Geometry check sheet. Reference: the model listing, model coordinates, mm. A direction names the side the tool comes from. Coordinates: 2 decimals unless noted, no trailing zeros. Loops run counter-clockwise (first coordinate to the right, second up) from the corner with the lowest first, then second, coordinate; pieces in that order, holes last. Notation, with made-up numbers: (-24, 44.25) - (5, 44.25) arc R17 cw to (5, 72.25) - close; hole circle Ø11 at (67, -4.75). An arc over 180 degrees is marked (long way). One line per item, written item: value.
from build123d import *

# Parameters (mm, degrees)
SKETCH_1_R          = 12.5
EXTRUDE_1_DEPTH     = 7.5
EXTRUDE_2_DEPTH     = 10
EXTRUDE_START       = -3
SKETCH_3_R          = 17
SKETCH_3_R_2        = 12.5
EXTRUDE_3_DEPTH     = 3
SKETCH_4_R          = 2.1000000000000005
CUT_EXTRUDE_1_DEPTH = 37.83761664386012
SKETCH_5_R          = 1.6000000000000003
CUT_EXTRUDE_2_DEPTH = 37.83761664386012
CUT_EXTRUDE_START   = -10
CUT_EXTRUDE_3_DEPTH = 10
SKETCH_7_R          = 17
SKETCH_7_R_2        = 12.500000000000004
EXTRUDE_4_DEPTH     = 0.5
SKETCH_8_R          = 15
SKETCH_8_R_2        = 12.499999999999996
EXTRUDE_5_DEPTH     = 11.5


# Read off the part's stored shape, not the designer's step: 凸台-拉伸2
with BuildPart() as part:
    # 草图1 → 凸台-拉伸1 (new, symmetric)
    with BuildSketch(Plane(origin=(0, 0, 0), x_dir=(1, 0, 0), z_dir=(0, 1, 0))):
        with Locations(Location((-1.39e-15, 1.39e-15, 0), (0, 0, 270))):
            Circle(SKETCH_1_R)
        with BuildLine():
            Line((6.600000000000003, -7.6000000000000005), (-6.599999999999996, -7.6000000000000005))
            ThreePointArc((-6.599999999999996, -7.6000000000000005), (-8.30710678118655, -8.307106781186542), (-7.599999999999978, -6.6000000000000005))
            Line((-7.599999999999996, -6.6000000000000005), (-7.599999999999996, 6.599999999999999))
            ThreePointArc((-7.599999999999978, 6.599999999999999), (-8.30710678118655, 8.30710678118654), (-6.599999999999996, 7.599999999999999))
            Line((-6.599999999999996, 7.599999999999999), (6.600000000000003, 7.599999999999999))
            ThreePointArc((6.600000000000002, 7.599999999999999), (7.600000000000003, 8.6), (8.600000000000005, 7.599999999999999))
            ThreePointArc((8.600000000000005, 7.599999999999999), (8.307106781186558, 6.892893218813457), (7.600000000000021, 6.599999999999998))
            Line((7.600000000000003, 6.599999999999999), (7.600000000000003, -6.6))
            ThreePointArc((7.600000000000021, -6.6), (8.307106781186558, -6.892893218813459), (8.600000000000003, -7.6000000000000005))
            ThreePointArc((8.600000000000003, -7.6000000000000005), (7.600000000000003, -8.600000000000001), (6.600000000000002, -7.6000000000000005))
        make_face(mode=Mode.SUBTRACT)
    extrude(amount=EXTRUDE_1_DEPTH, both=True)

    # 凸台-拉伸2 outline → 凸台-拉伸2 (add)
    with BuildSketch(Plane.XZ.offset(7.5)):
        with BuildLine():
            Line((10.6, -6.62495283), (10.6, 6.62495283))
            ThreePointArc((10.6, 6.62495283), (8.838834765, 8.838834765), (6.62495283, 10.6))
            Line((6.62495283, 10.6), (-6.62495283, 10.6))
            ThreePointArc((-6.62495283, 10.6), (-8.838834765, 8.838834765), (-10.6, 6.62495283))
            Line((-10.6, 6.62495283), (-10.6, -6.62495283))
            ThreePointArc((-10.6, -6.62495283), (-8.838834765, -8.838834765), (-6.62495283, -10.6))
            Line((-6.62495283, -10.6), (6.62495283, -10.6))
            ThreePointArc((6.62495283, -10.6), (8.838834765, -8.838834765), (10.6, -6.62495283))
        make_face()
        with BuildLine():
            ThreePointArc((-6.6, -7.6), (-8.307106781, -8.307106781), (-7.6, -6.6))
            Line((-7.6, -6.6), (-7.6, 6.6))
            ThreePointArc((-7.6, 6.6), (-8.307106781, 8.307106781), (-6.6, 7.6))
            Line((-6.6, 7.6), (6.6, 7.6))
            ThreePointArc((6.6, 7.6), (8.307106781, 8.307106781), (7.6, 6.6))
            Line((7.6, 6.6), (7.6, -6.6))
            ThreePointArc((7.6, -6.6), (8.307106781, -8.307106781), (6.6, -7.6))
            Line((6.6, -7.6), (-6.6, -7.6))
        make_face(mode=Mode.SUBTRACT)
    extrude_2 = extrude(amount=EXTRUDE_2_DEPTH)

    # 镜向1: 凸台-拉伸2 across plane
    add(extrude_2.mirror(Plane.ZX))

    # 草图3 → 凸台-拉伸3 (add)
    with BuildSketch(Plane.XZ.offset(7.5).offset(EXTRUDE_START)):
        with Locations(Location((0, 0, 0), (0, 0, 270))):
            Circle(SKETCH_3_R)
        with Locations(Location((0, 0, 0), (0, 0, 270))):
            Circle(SKETCH_3_R_2, mode=Mode.SUBTRACT)
    extrude(amount=EXTRUDE_3_DEPTH)

    # 草图4 → 切除-拉伸1 (cut, through all)
    with BuildSketch(Plane.XY.offset(10.600000000000001)):
        with Locations((-8.7e-16, -12.5)):
            Circle(SKETCH_4_R)
    extrude(amount=-CUT_EXTRUDE_1_DEPTH, mode=Mode.SUBTRACT)

    # 草图5 → 切除-拉伸2 (cut, through all)
    with BuildSketch(Plane(origin=(10.6, 0, 0), x_dir=(0, 0, -1), z_dir=(1, 0, 0))):
        with Locations((1.73e-15, 12.5)):
            Circle(SKETCH_5_R)
    extrude(amount=-CUT_EXTRUDE_2_DEPTH, mode=Mode.SUBTRACT)

    # 草图6 → 切除-拉伸3 (cut)
    with BuildSketch(Plane.XZ.offset(17.5).offset(CUT_EXTRUDE_START)):
        with BuildLine():
            Line((10.599999999999996, -6.624952830020757), (10.6, 6.624952830020752))
            ThreePointArc((10.6, 6.624952830020752), (8.83883476483184, 8.838834764831846), (6.6249528300207485, 10.600000000000001))
            Line((6.6249528300207485, 10.600000000000001), (-6.624952830020753, 10.600000000000001))
            ThreePointArc((-6.624952830020753, 10.600000000000001), (-8.838834764831846, 8.838834764831844), (-10.6, 6.624952830020758))
            Line((-10.6, 6.624952830020758), (-10.6, -6.624952830020761))
            ThreePointArc((-10.6, -6.624952830020761), (-8.83883476483185, -8.838834764831843), (-6.624952830020767, -10.599999999999994))
            Line((-6.624952830020767, -10.599999999999994), (6.624952830020759, -10.599999999999998))
            ThreePointArc((6.624952830020759, -10.599999999999998), (8.838834764831844, -8.838834764831844), (10.599999999999996, -6.624952830020757))
        make_face()
    extrude(amount=CUT_EXTRUDE_3_DEPTH, mode=Mode.SUBTRACT)

    # 草图7 → 凸台-拉伸4 (add)
    with BuildSketch(Plane(origin=(0, -4.5, 0), x_dir=(1, 0, 0), z_dir=(0, 1, 0))):
        with Locations(Location((0, 0, 0), (0, 0, 90))):
            Circle(SKETCH_7_R)
        with Locations(Location((0, 0, 0), (0, 0, 122.005199861))):
            Circle(SKETCH_7_R_2, mode=Mode.SUBTRACT)
    extrude(amount=EXTRUDE_4_DEPTH)

    # 草图8 → 凸台-拉伸5 (add)
    with BuildSketch(Plane(origin=(0, -4, 0), x_dir=(1, 0, 0), z_dir=(0, 1, 0))):
        with Locations(Location((0, 0, 0), (0, 0, 270))):
            Circle(SKETCH_8_R)
        Circle(SKETCH_8_R_2, mode=Mode.SUBTRACT)
    extrude(amount=EXTRUDE_5_DEPTH)


solid = part.part
(1) Release check for a two-part mould opening along Z. For faces 5 (the face through (9.121, 14.086, 0.208)), 6 (the face through (8.87, 12.43, 8.81)), 7 (the face through (0, -7.5, 8)) record: pulls with the +Z half, pulls with the -Z half, needs draft (parallel to the pull), parting line crosses it, or undercut.
Reply:
face 5: undercut
face 6: pulls with the +Z half
face 7: needs draft
(2) Cross-section at C-C on z = 2.5. Record the cut outline in (x, y).
Reply:
outline: (-16.82, -7.5) - (-7.6, -7.5) - (-7.6, 17.5) - (-10.6, 17.5) - (-10.6, 7.5) - (-14.79, 7.5) - (-14.79, -4) - (-16.82, -4) - close; (7.6, -7.5) - (16.82, -7.5) - (16.82, -4) - (14.79, -4) - (14.79, 7.5) - (10.6, 7.5) - (10.6, 17.5) - (7.6, 17.5) - close
(3) Cross-section at A-A on x = 0. Record the cut outline in (y, z).
Reply:
outline: (-7.5, -17) - (-4, -17) - (-4, -15) - (7.5, -15) - (7.5, -10.6) - (17.5, -10.6) - (17.5, -7.6) - (-7.5, -7.6) - close; (-7.5, 7.6) - (17.5, 7.6) - (17.5, 10.6) - (7.5, 10.6) - (7.5, 15) - (-4, 15) - (-4, 17) - (-7.5, 17) - close
(4) Cross-section at D-D on y = 4.25. Record the cut outline in (x, z).
Reply:
outline: circle Ø30 at (0, 0); hole (-7.6, -6.6) arc R1 ccw (long way) to (-6.6, -7.6) - (6.6, -7.6) arc R1 ccw (long way) to (7.6, -6.6) - (7.6, 6.6) arc R1 ccw (long way) to (6.6, 7.6) - (-6.6, 7.6) arc R1 ccw (long way) to (-7.6, 6.6) - close
(5) Go/stop test with flat-tipped pins: pin 1 Ø3 at (x, y) = (3, 12.5) entering from -Z; pin 2 Ø8 at (y, z) = (2.5, 9) entering from -X; pin 3 Ø3 at (y, z) = (12, -3) entering from +X; pin 4 Ø1 at (x, y) = (12.5, 12.5) entering from +Z. Record where each tip stops, or that it passes through.
Reply:
pin 1: z = -10.6
pin 2: x = -14.14
pin 3: x = 10.6
pin 4: through
(6) Material ranges on probe 1 along Z at (x, y) = (3, 14); probe 2 along Z at (x, y) = (-3.5, -0.75), recorded low to high. Write a range as from..to.
Reply:
probe 1: -10.6..-7.6, 7.6..10.6
probe 2: -14.59..-7.6, 7.6..14.59
(7) Cross-section at B-B on y = 12.5. Record the cut outline in (x, z).
Reply:
outline: (-10.6, -6.62) arc R12.5 ccw to (-6.62, -10.6) - (6.62, -10.6) arc R12.5 ccw to (10.6, -6.62) - (10.6, -1.6) - (7.6, -1.6) - (7.6, -6.6) arc R1 cw (long way) to (6.6, -7.6) - (-6.6, -7.6) arc R1 cw (long way) to (-7.6, -6.6) - (-7.6, -1.6) - (-10.6, -1.6) - close; (-10.6, 1.6) - (-7.6, 1.6) - (-7.6, 6.6) arc R1 cw (long way) to (-6.6, 7.6) - (6.6, 7.6) arc R1 cw (long way) to (7.6, 6.6) - (7.6, 1.6) - (10.6, 1.6) - (10.6, 6.62) arc R12.5 ccw to (6.62, 10.6) - (-6.62, 10.6) arc R12.5 ccw to (-10.6, 6.62) - close
(8) Access from +Z, -Z, +X, -X, +Y, -Y to the whole of each face (thin tool, end or side, straight path). Record for faces 1 (the face through (10.6, 14, -2)), 2 (the face through (0, 12, -10.6)), 3 (the face through (-11, 7.5, 0)), 4 (the face through (7.6, 5, 0)).
Reply:
face 1: +Z, -Z, +X, +Y
face 2: -Z, +X, -X, +Y
face 3: +Y
face 4: +Y, -Y
